from build123d import *

# Parameters (mm, degrees)
F0_W     = 76.2
F0_H     = 76.2
F1_DEPTH = 38.1
F3_DEPTH = 76.201


with BuildPart() as f1:
    # F0 (on Front) → F1 (new body, symmetric)
    with BuildSketch(Plane.XZ):
        Rectangle(F0_W, F0_H)
    extrude(amount=F1_DEPTH, both=True)

    # F2 (on face) → F3 (cut, through all)
    with BuildSketch(Plane.XZ.offset(38.1)):
        Polygon((0, 21.997045), (-12.7, 0), (12.7, 0), align=None)
    extrude(amount=-F3_DEPTH, mode=Mode.SUBTRACT)


solid = f1.part
Verification items for the finished model (mm, model axes). A direction names the side the tool comes from. Coordinates: 2 decimals unless noted, no trailing zeros. Order: outer loops, then holes, each group sorted by start corner. A loop starts at its lowest first (then second) coordinate and runs counter-clockwise, first axis right, second up. Notation, with made-up numbers: M -14.5,25.25 L 16.5,25.25 A19 cw 16.5,39.25 Z; hole C 64,7 d5. An arc over 180 degrees is marked long. Return JSON: item names as keys, results as strings.
1) Cross-section at B-B, the plane x = 7.5. Record the boundary of the cut face in (y, z), and give its area (3 significant figures).
Answer list:
{"outline": "M -38.1,-38.1 L 38.1,-38.1 L 38.1,0 L -38.1,0 Z; M -38.1,9.01 L 38.1,9.01 L 38.1,38.1 L -38.1,38.1 Z", "area": "5,120 mm2"}
2) Release check for a two-part mould opening along X. For faces 1 (the flat face through (-1, -38.1, -8)), 2 (the flat face through (6.44, -0.53, 10.84)), 3 (the flat face through (-38.1, -1, -1)) record: +X half, -X half, draft (parallel to the pull), parting line (faces both ways), or undercut.
Answer list:
{"face 1": "draft", "face 2": "undercut", "face 3": "-X half"}
3) Access from +Z, -Z, +X, -X, +Y, -Y to the whole of each face (thin tool, end or side, straight path). Record for faces 4 (the flat face through (-6.261, -0.533, 11.153)), 5 (the flat face through (-1, 38.1, -8)).
Answer list:
{"face 4": "+Y, -Y", "face 5": "+Z, -Z, +X, -X, +Y"}
4) Cross-section at A-A, the plane y = -4. Record the boundary of the cut face in (x, z).
Answer list:
{"outline": "M -38.1,-38.1 L 38.1,-38.1 L 38.1,38.1 L -38.1,38.1 Z; hole M -12.7,0 L 12.7,0 L 0,22 Z"}
5) Thickness scan on L1, parallel to X at y = -31, z = 12; L2, parallel to X at y = 30.5, z = 14; L3, parallel to Z at x = -8, y = -13. Record the ranges inside material, lowest first. Write a range as [from, to].
Answer list:
{"L1": "[-38.1, -5.77], [5.77, 38.1]", "L2": "[-38.1, -4.62], [4.62, 38.1]", "L3": "[-38.1, 0], [8.14, 38.1]"}
6) Cross-section at C-C, the plane z = 6.5. Record the boundary of the cut face in (x, y).
Answer list:
{"outline": "M -38.1,-38.1 L -8.95,-38.1 L -8.95,38.1 L -38.1,38.1 Z; M 8.95,-38.1 L 38.1,-38.1 L 38.1,38.1 L 8.95,38.1 Z"}
